Drawing for the job (mm, zero at the part's lowest x, y, z). A direction names the side the tool comes from. Give positions to 0.01 mm unless a question says otherwise; leave off trailing zeros. Order: outer loops, then holes, each group sorted by start corner. A loop starts at its lowest first (then second) coordinate and runs counter-clockwise, first axis right, second up. Notation, with made-up numbers: (39, 62.25) - (55, 62.25) arc R11 ccw to (55, 76.25) - close; hole circle Ø6 at (86, 66). An arc over 180 degrees is marked (long way). Write each question's results on one line, items separated by ' | '. Start each with the question number.
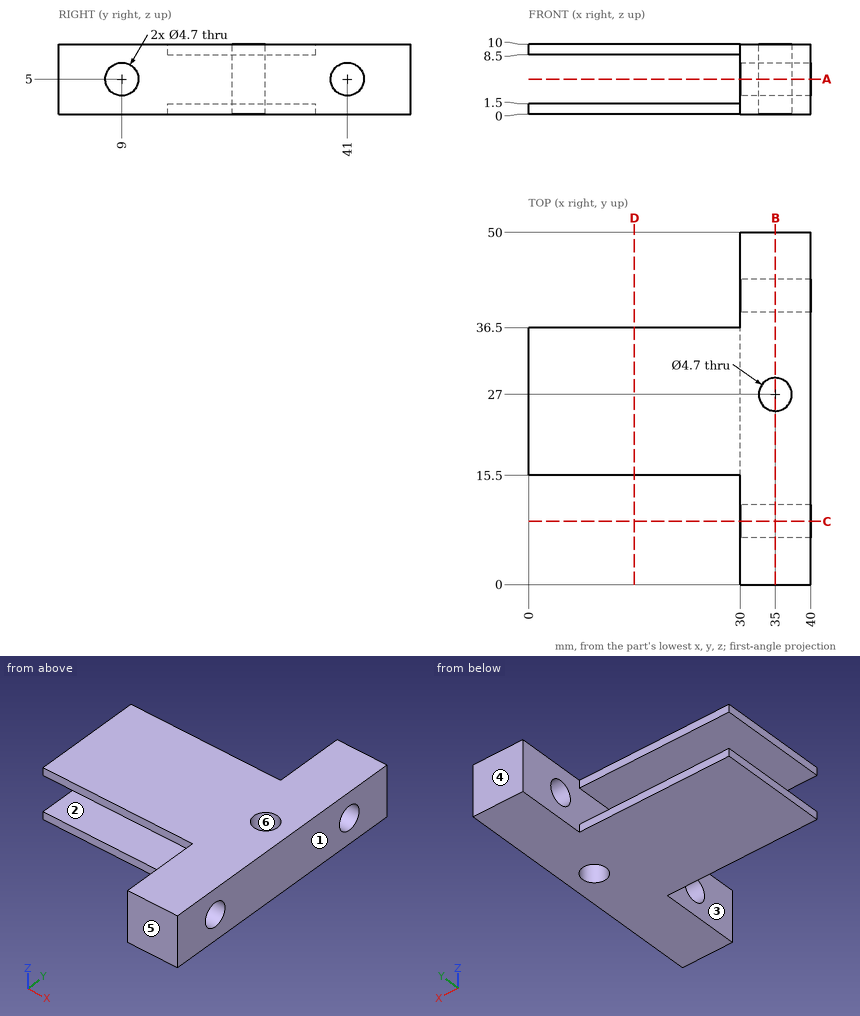
Item 1: Two-plate mould, pull along Y, no slides. Class the marked faces 3, 4, 5 and 6: +Y half, -Y half, draft (parallel to the pull), parting line (faces both ways), or undercut.
Item 2: Cut at B-B, the plane x = 35. List the corners of the cut face in (y, z).
Item 3: Cut at C-C, the plane y = 9. List the corners of the cut face in (x, z), then the cut area to 3 significant figures.
Item 4: Cut at D-D, the plane x = 15. List the corners of the cut face in (y, z).
Item 5: Which spindle directions (+Z, -Z, +X, -X, +Y, -Y) get a long thin tool onto all of the face, cutting with end or side? Do the marked faces 1 and 2. Say none if no direction does.
Item 6: Flat gauge pins, fed straight in: pin 1 Ø23 at (x, y) = (21, 25.5) entering from -Z; pin 2 Ø0.8 at (x, z) = (14, 0.5) entering from +Y; pin 3 Ø5 at (x, z) = (15.5, 8.5) entering from -Y. Where does each tip first touch, or does it go through?
Item 7: Probe line 1 along Z through (x, y) = (22.5, 18); line 2 along Y through (x, z) = (38, 5); line 3 along Y through (x, z) = (36.25, 5). List the from-to ranges inside material, lowest first. Write a range as from..to.
Item 8: Cut at A-A, the plane z = 5. List the corners of the cut face in (x, y).
Values found:
1) face 3: draft | face 4: +Y half | face 5: -Y half | face 6: undercut
2) outline: (0, 0) - (24.65, 0) - (24.65, 10) - (0, 10) - close; (29.35, 0) - (50, 0) - (50, 10) - (29.35, 10) - close; hole circle Ø4.7 at (9, 5); hole circle Ø4.7 at (41, 5)
3) outline: (30, 0) - (40, 0) - (40, 2.65) - (30, 2.65) - close; (30, 7.35) - (40, 7.35) - (40, 10) - (30, 10) - close | area: 53.0 mm2
4) outline: (15.5, 0) - (36.5, 0) - (36.5, 1.5) - (15.5, 1.5) - close; (15.5, 8.5) - (36.5, 8.5) - (36.5, 10) - (15.5, 10) - close
5) face 1: +Z, -Z, +X, +Y, -Y | face 2: -X, +Y, -Y
6) pin 1: stops at z = 0 | pin 2: stops at y = 36.5 | pin 3: stops at y = 15.5
7) line 1: z = 0..1.5, 8.5..10 | line 2: y = 0..6.65, 11.35..38.65, 43.35..50 | line 3: y = 0..6.65, 11.35..25.01, 28.99..38.65, 43.35..50
8) outline: (30, 0) - (40, 0) - (40, 6.65) - (30, 6.65) - close; (30, 11.35) - (40, 11.35) - (40, 38.65) - (30, 38.65) - close; (30, 43.35) - (40, 43.35) - (40, 50) - (30, 50) - close; hole circle Ø4.7 at (35, 27)
